Geometry check sheet. Reference: the model listing, model coordinates, mm. A direction names the side the tool comes from. Round coordinates to 2 decimals unless told otherwise and drop trailing zeros. Loops run counter-clockwise (first coordinate to the right, second up) from the corner with the lowest first, then second, coordinate; pieces in that order, holes last.
```python
from build123d import *

# Parameters (mm, degrees)
ESBO_O1_R                  = 30
RESSALTO_EXTRUS_O1_DEPTH   = 2
ESBO_O2_R                  = 30
ESBO_O2_R_2                = 11.5
CORTE_EXTRUS_O6_DEPTH      = 0.35
ESBO_O9_R                  = 11.5
CORTE_EXTRUS_O7_DEPTH      = 37
CORTE_EXTRUS_O7_DEPTH_BACK = 12.35
FILETE2_R                  = 0.25
ESBO_O10_R                 = 15.5
CORTE_EXTRUS_O8_DEPTH      = 0.35


with BuildPart() as part:
    # Esboço1 → Ressalto-extrusão1 (new body)
    with BuildSketch(Plane.XY):
        Circle(ESBO_O1_R)
    extrude(amount=RESSALTO_EXTRUS_O1_DEPTH)

    # Esboço2 → Corte-extrusão6 (cut)
    with BuildSketch(Plane(origin=(0, 0, 0), x_dir=(-1, 0, 0), z_dir=(0, 0, -1))):
        Circle(ESBO_O2_R)
        Circle(ESBO_O2_R_2, mode=Mode.SUBTRACT)
        with BuildLine():
            Line((-17.462157831, -20.593033868), (-9.611804273, -12.159902081))
            ThreePointArc((-9.611804273, -12.159902081), (-5.674511924, -14.423935469), (-1.25, -15.449514555))
            Line((-1.25, -15.449514555), (-1.25, -26.971049294))
            ThreePointArc((-1.25, -26.971049294), (-9.884633674, -25.125565011), (-17.462157831, -20.593033868))
        make_face(mode=Mode.SUBTRACT)
        with BuildLine():
            Line((1.25, -26.971049294), (1.25, -15.449514555))
            ThreePointArc((1.25, -15.449514555), (6.35222208, -14.138573996), (10.720700103, -11.194489238))
            Line((10.720700103, -11.194489238), (19.334766503, -18.845869687))
            ThreePointArc((19.334766503, -18.845869687), (11.065161043, -24.628483735), (1.25, -26.971049294))
        make_face(mode=Mode.SUBTRACT)
        with BuildLine():
            Line((-26.971049294, -1.25), (-15.449514555, -1.25))
            ThreePointArc((-15.449514555, -1.25), (-14.211748443, -6.186776721), (-11.441667216, -10.456493261))
            Line((-11.441667216, -10.456493261), (-19.292020774, -18.889625048))
            ThreePointArc((-19.292020774, -18.889625048), (-24.755948901, -10.7769659), (-26.971049294, -1.25))
        make_face(mode=Mode.SUBTRACT)
        with BuildLine():
            Line((-26.971049294, 1.25), (-15.449514555, 1.25))
            ThreePointArc((-15.449514555, 1.25), (-14.489180857, 5.50578224), (-12.380934748, 9.325366201))
            Line((-12.380934748, 9.325366201), (-20.995001147, 16.97674665))
            ThreePointArc((-20.995001147, 16.97674665), (-25.239218268, 9.590717451), (-26.971049294, 1.25))
        make_face(mode=Mode.SUBTRACT)
        with BuildLine():
            Line((20.995001147, -16.976746651), (12.380934747, -9.325366201))
            ThreePointArc((12.380934747, -9.325366201), (14.489180857, -5.50578224), (15.449514555, -1.25))
            Line((15.449514555, -1.25), (26.971049294, -1.25))
            ThreePointArc((26.971049294, -1.25), (25.239218268, -9.590717451), (20.995001147, -16.976746651))
        make_face(mode=Mode.SUBTRACT)
        with BuildLine():
            Line((15.449514555, 1.25), (26.971049294, 1.25))
            ThreePointArc((26.971049294, 1.25), (24.755948901, 10.776965901), (19.292020774, 18.889625048))
            Line((19.292020774, 18.889625048), (11.441667216, 10.456493261))
            ThreePointArc((11.441667216, 10.456493261), (14.211748443, 6.186776721), (15.449514555, 1.25))
        make_face(mode=Mode.SUBTRACT)
        with BuildLine():
            Line((9.611804273, 12.159902081), (17.462157831, 20.593033868))
            ThreePointArc((17.462157831, 20.593033868), (9.884633674, 25.125565011), (1.25, 26.971049294))
            Line((1.25, 26.971049294), (1.25, 15.449514555))
            ThreePointArc((1.25, 15.449514555), (5.674511924, 14.423935469), (9.611804273, 12.159902081))
        make_face(mode=Mode.SUBTRACT)
        with BuildLine():
            Line((-1.25, 15.449514555), (-1.25, 26.971049294))
            ThreePointArc((-1.25, 26.971049294), (-11.065161043, 24.628483735), (-19.334766503, 18.845869687))
            Line((-19.334766503, 18.845869687), (-10.720700104, 11.194489238))
            ThreePointArc((-10.720700104, 11.194489238), (-6.35222208, 14.138573996), (-1.25, 15.449514555))
        make_face(mode=Mode.SUBTRACT)
    extrude(amount=-CORTE_EXTRUS_O6_DEPTH, mode=Mode.SUBTRACT)

    # Esboço9 → Corte-extrusão7 (cut, two sides)
    with BuildSketch(Plane(origin=(0, 0, 0), x_dir=(-1, 0, 0), z_dir=(0, 0, -1))) as corte_extrus_o7_sk:
        Circle(ESBO_O9_R)
    extrude(amount=CORTE_EXTRUS_O7_DEPTH, mode=Mode.SUBTRACT)
    extrude(corte_extrus_o7_sk.sketch, amount=-CORTE_EXTRUS_O7_DEPTH_BACK, mode=Mode.SUBTRACT)

    # Filete2
    filete2_edges = [part.edges().sort_by_distance(p)[0] for p in [
        (-30, 0, 0.35),
        (-30, 0, 2),
    ]]
    fillet(filete2_edges, radius=FILETE2_R)

    # Esboço10 → Corte-extrusão8 (cut)
    with BuildSketch(Plane.XY.offset(2)):
        Circle(ESBO_O10_R)
    extrude(amount=-CORTE_EXTRUS_O8_DEPTH, mode=Mode.SUBTRACT)


solid = part.part
```
1) Gauge pin test, flat ends, axial feed: pin 1 (2 mm diameter, centred on x = 6, y = 7, fed in from +Z); pin 2 (1 mm diameter, centred on x = -10, z = 1.5, fed in from -Y). Record the tip position at first contact, or that the pin passes through.
Report:
pin 1: passes through
pin 2: stops at y = -28.46
2) Sectioned sample at A-A, the plane y = 0. Record the cut outline in (x, z), then the cut area to 3 significant figures.
Report:
outline: (-30, 0.6) arc R0.25 ccw to (-29.75, 0.35) - (-11.5, 0.35) - (-11.5, 1.65) - (-15.5, 1.65) - (-15.5, 2) - (-29.75, 2) arc R0.25 ccw to (-30, 1.75) - close; (11.5, 0.35) - (29.75, 0.35) arc R0.25 ccw to (30, 0.6) - (30, 1.75) arc R0.25 ccw to (29.75, 2) - (15.5, 2) - (15.5, 1.65) - (11.5, 1.65) - close
area: 58.2 mm2
3) Sectioned sample at C-C, the plane z = 1.3. Record the cut outline in (x, y).
Report:
outline: circle Ø60 at (0, 0); hole circle Ø23 at (0, 0)
4) Access from +Z, -Z, +X, -X, +Y, -Y to the whole of each face (thin tool, end or side, straight path). Record for faces 1 (the face through (-25.28, -9.48, 0.17)), 2 (the face through (-5.615, 14.447, 0.173)), 3 (the face through (20, 7, 0)).
Report:
face 1: -Z, -X, -Y
face 2: -Z
face 3: -Z, +X, -X, +Y, -Y
5) Mould release check, pull along Y, two halves, no side actions. Record for faces 4 (the face through (9.77, -25.17, 0.17)), 5 (the face through (-19, 8, 0)), 6 (the face through (15.3, -14.6, 0.2)): +Y half, -Y half, draft (parallel to the pull), parting line (faces both ways), or undercut.
Report:
face 4: -Y half
face 5: draft
face 6: undercut
6) Scan lines: line 1 along Y through (x, z) = (0, 0.9); line 2 along Z through (x, y) = (18.5, -19); line 3 along X through (y, z) = (-3, 1.2). Record each from-to range of solid material in increasing order.
Report:
line 1: y = -30 to -11.5, 11.5 to 30
line 2: z = 0.35 to 2
line 3: x = -29.85 to -11.1, 11.1 to 29.85
